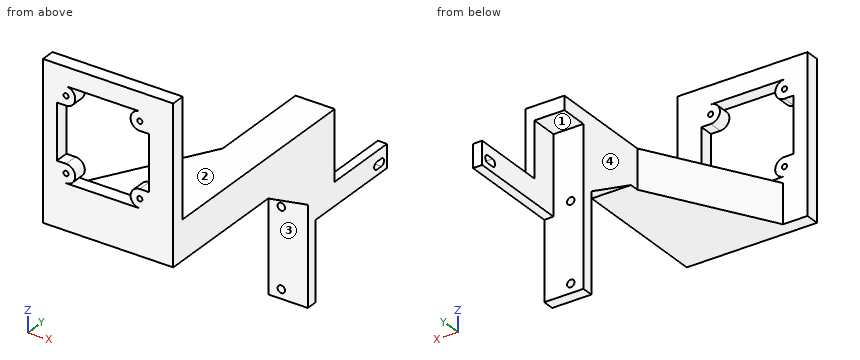
Autodesk Inventor part; units mm, degrees
ref_plane "YZ Plane" through (0, 0, 0) normal (1, 0, 0) x (0, 1, 0)
ref_plane "XZ Plane" through (0, 0, 0) normal (0, 1, 0) x (-1, 0, 0)
ref_plane "XY Plane" through (0, 0, 0) normal (0, 0, 1) x (1, 0, 0)
sketch "Sketch1" plane through (0, 0, 0) normal (0, 1, 0) x (-1, 0, 0)
  line L0 (0, 0) -> (13, 0)
  line L1 (13, 0) -> (13, -44)
  line L2 (13, -44) -> (0, -44)
  line L3 (0, -44) -> (0, 0)
  line L4 (13, 0) -> (13, -6)
  line L5 (13, -6) -> (7.5, -6)
  line L6 (7.5, -6) -> (7.5, -40)
  circle A0 centre (7.5, -6) radius 1.6
  circle A1 centre (7.5, -40) radius 1.6
  dimension "d0" = 13
  dimension "d1" = 44
  dimension "d2" = 6
  dimension "d3" = 5.5
  dimension "d4" = 34
  dimension "d5" = 3.2
  dimension "d6" = 3.2
extrude "Extrusion1" add sketch "Sketch1" along normal blind 5
sketch "Sketch2" plane through (0, 0, 0) normal (1, 0, 0) x (0, 0, -1)
  line L0 (0, 5) -> (44, 5)
  line L1 (0, 5) -> (44, 5)
  line L2 (44, 5) -> (44, 50)
  line L3 (44, 50) -> (0, 50)
  line L4 (0, 50) -> (0, 5)
  line L5 (0, 0) -> (44, 0)
  line L6 (44, 0) -> (44, 5)
  line L7 (44, 5) -> (0, 5)
  line L8 (0, 5) -> (0, 0)
  line L9 (0, 50) -> (10, 50)
  line L10 (10, 50) -> (10, 5)
  line L11 (10, 5) -> (0, 5)
  line L12 (0, 5) -> (0, 50)
  dimension "d9" = 44
  dimension "d10" = 45
  dimension "d11" = 10
extrude "Extrusion2" add sketch "Sketch2" along normal blind 4 contours L4 L3 L10 L0 | L0 L6 L5 L8
sketch "Sketch3" plane through (4, 0, 0) normal (1, 0, 0) x (0, 0, -1)
  line L0 (44, 5) -> (10, 5)
  line L1 (10, 5) -> (10, 45)
  line L2 (10, 5) -> (10, 50)
  line L3 (0, 50) -> (0, 5)
  line L4 (0, 45) -> (4.4, 45)
  line L5 (6, 45) -> (6, 46.5)
  line L6 (6, 45) -> (6, 43.5)
  line L7 (4.4, 46.5) -> (4.4, 43.5)
  line L8 (7.6, 46.5) -> (7.6, 43.5)
  arc A0 (5.4432, 45) -> (6, 44.9) centre (6, 46.5) ccw
  arc A1 (6.5568, 45) -> (4.4, 46.5) centre (6, 46.5) ccw
  line L9 (10, 45) -> (6.5568, 45)
  line L10 (5.4432, 45) -> (0, 45)
  arc A2 (6, 45.1) -> (5.4432, 45) centre (6, 43.5) ccw
  arc A3 (4.4, 43.5) -> (7.6, 43.5) centre (6, 43.5) ccw
  point P0 (0, 0)
  dimension "d14" = 40
  dimension "d15" = 6
  dimension "d16" = 1.5
  dimension "d17" = 1.5
extrude "Extrusion3" cut sketch "Sketch3" against normal blind 4 contours L6 A0 A2 L5 | A1 L9 L8 A3 L7 | L8 L9 A1
sketch "Sketch4" plane through (-13, 0, 0) normal (0, 0, 1) x (1, 0, 0)
  line L0 (0, 0) -> (17, 0)
  line L1 (17, 0) -> (17, 5)
  line L2 (0, 0) -> (17, 0)
  line L3 (17, 0) -> (17, 5)
  line L4 (17, 5) -> (0, 5)
  line L5 (0, 5) -> (0, 0)
  line L6 (13, 50) -> (13, 5)
  line L7 (17, 0) -> (13, 0)
  line L8 (13, 0) -> (13, 17)
  line L9 (13, 17) -> (17, 17)
  line L10 (17, 17) -> (17, 0)
  dimension "d22" = 17
extrude "Extrusion4" add sketch "Sketch4" along normal blind 30
sketch "Sketch5" plane through (0, 0, 0) normal (0, -1, 0) x (1, 0, 0)
  line L0 (-13, -44) -> (-13, 30)
  line L1 (-13, 30) -> (4, 30)
  line L2 (4, 30) -> (4, 13)
  line L3 (4, 13) -> (-13, 13)
  line L4 (-13, 13) -> (-13, 30)
  point P0 (0, 0)
  dimension "d25" = 17
  dimension "d26" = 17
extrude "Extrusion5" add sketch "Sketch5" along normal blind 85
sketch "Sketch7" plane through (0, -85, 0) normal (0, -1, 0) x (1, 0, 0)
  line L0 (4, 13) -> (-13, 13)
  line L1 (0, 30) -> (0, -10)
  line L2 (0, 13) -> (0, 30)
  line L3 (0, 30) -> (0, 52.6)
  circle A0 centre (-36, 52.6) radius 9
  line L4 (-36, 52.6) -> (-36, 36.6)
  line L5 (-36, 36.6) -> (-20, 36.6)
  line L6 (-36, 52.6) -> (-36, 68.6)
  line L7 (-36, 68.6) -> (-52, 68.6)
  line L8 (-52, 68.6) -> (-20, 68.6)
  line L9 (-20, 68.6) -> (-20, 36.6)
  line L10 (-20, 36.6) -> (-52, 36.6)
  line L11 (-52, 36.6) -> (-52, 68.6)
  circle A1 centre (-20, 68.6) radius 1.1
  circle A2 centre (-20, 36.6) radius 1.1
  circle A3 centre (-52, 36.6) radius 1.1
  circle A4 centre (-52, 68.6) radius 1.1
  circle A5 centre (-20, 68.6) radius 4
  circle A6 centre (-20, 36.6) radius 4
  line L12 (-52, 65.6) -> (-52, 70.6)
  line L13 (-52, 36.6) -> (-52, 42.6)
  circle A7 centre (-52, 68.6) radius 4
  circle A8 centre (-52, 36.6) radius 4
  point P0 (0, 0)
  point P1 (-20, 64.6)
  point P2 (-20, 40.6)
  dimension "d29" = 22.6
  dimension "d31" = 18
  dimension "d32" = 16
  dimension "d33" = 16
  dimension "d34" = 16
  dimension "d35" = 16
  dimension "d36" = 2.2
  dimension "d37" = 2.2
  dimension "d39" = 2.2
  dimension "d40" = 8
  dimension "d43" = 8
  dimension "d49" = 8
  dimension "d50" = 8
sketch "Sketch14" plane through (0, -85, 0) normal (0, -1, 0) x (1, 0, 0)
  line L0 (4, 13) -> (4, 30)
  line L1 (4, 13) -> (4, 52.6)
  line L2 (4, 52.6) -> (-26.5, 52.6)
  line L3 (-26.5, 52.6) -> (-26.5, 36.6)
  line L4 (-26.5, 36.6) -> (-10.5, 36.6)
  line L5 (-26.5, 52.6) -> (-42.5, 52.6)
  line L6 (-42.5, 52.6) -> (-42.5, 68.6)
  line L7 (-42.5, 68.6) -> (-10.5, 68.6)
  line L8 (-10.5, 68.6) -> (-10.5, 36.6)
  line L9 (-10.5, 36.6) -> (-42.5, 36.6)
  line L10 (-42.5, 36.6) -> (-42.5, 68.6)
  circle A0 centre (-42.5, 68.6) radius 1.1
  circle A1 centre (-10.5, 68.6) radius 1.1
  circle A2 centre (-10.5, 36.6) radius 1.1
  circle A3 centre (-42.5, 36.6) radius 1.1
  circle A4 centre (-42.5, 68.6) radius 4
  circle A5 centre (-10.5, 68.6) radius 4
  circle A6 centre (-10.5, 36.6) radius 4
  circle A7 centre (-42.5, 36.6) radius 4
  point P0 (0, 0)
  dimension "d91" = 39.6
  dimension "d92" = 30.5
  dimension "d93" = 16
  dimension "d94" = 16
  dimension "d95" = 16
  dimension "d96" = 16
  dimension "d97" = 2.2
  dimension "d98" = 2.2
  dimension "d99" = 2.2
  dimension "d100" = 2.2
  dimension "d101" = 8
  dimension "d102" = 8
  dimension "d103" = 8
  dimension "d104" = 8
extrude "Extrusion14" add sketch "Sketch14" against normal blind 6 contours A5 L7 A1 L8 | L8 A1 L7 A5 | A6 L4 A2 L8 | L8 A2 L4 A6 | A7 L10 A3 L9 | L9 A3 L10 A7 | A4 L7 A0 L6 | L6 A0 L7 A4
sketch "Sketch15" plane through (-10.5, -85, 68.6) normal (0, -1, 0) x (1, 0, 0)
  circle A0 centre (0, 0) radius 4
  line L0 (0, 4) -> (10, 4)
  line L1 (10, 4) -> (10, -4)
  line L2 (10, -4) -> (0, -4)
  line L3 (0, -4) -> (0, 4)
  circle A1 centre (0, -32) radius 4
  line L4 (0, -28) -> (10, -28)
  line L5 (10, -28) -> (10, -36)
  line L6 (10, -36) -> (0, -36)
  line L7 (0, -36) -> (0, -28)
  circle A2 centre (-32, -32) radius 4
  line L8 (-32, -36) -> (-42, -36)
  line L9 (-42, -36) -> (-42, -28)
  line L10 (-42, -28) -> (-32, -28)
  line L11 (-32, -28) -> (-32, -36)
  circle A3 centre (-32, 0) radius 4
  line L12 (-32, -4) -> (-42, -4)
  line L13 (-42, -4) -> (-42, 4)
  line L14 (-42, 4) -> (-32, 4)
  line L15 (-32, 4) -> (-32, -4)
  line L16 (-42, 4) -> (-36, 4)
  line L17 (-36, 4) -> (-36, -36)
  line L18 (-36, -36) -> (-42, -36)
  line L19 (-42, -36) -> (-42, 4)
  line L20 (10, 4) -> (4, 4)
  line L21 (4, 4) -> (4, -36)
  line L22 (4, -36) -> (10, -36)
  line L23 (10, -36) -> (10, 4)
  point P0 (10.5, -68.6)
  point P1 (-36, -4)
  point P2 (-32, 4)
  point P3 (-42, -4)
  point P4 (-36, -28)
  point P5 (0, -4)
  point P6 (4, -4)
  point P7 (4, -28)
  point P8 (10, -4)
  dimension "d107" = 10
  dimension "d108" = 8
  dimension "d109" = 10
  dimension "d110" = 8
  dimension "d111" = 10
  dimension "d112" = 8
  dimension "d113" = 10
  dimension "d114" = 8
  dimension "d115" = 6
  dimension "d116" = 6
extrude "Extrusion15" add sketch "Sketch15" against normal blind 6 contours L21 L2 A0 | A0 L0 L21 | L21 L0 L1 L2 | L2 L23 L4 L21 | L21 A1 L4 | L4 L5 L6 L21 | L21 L6 A1 | A2 L17 L10 | L8 L17 A2 | L17 L8 L9 L10 | L10 L19 L12 L17 | L17 A3 L12 | L12 L13 L14 L17 | L17 L14 A3
sketch "Sketch16" plane through (0, -85, 0) normal (0, -1, 0) x (1, 0, 0)
  line L0 (-0.5, 72.6) -> (-0.5, 32.6)
  line L1 (-0.5, 72.6) -> (-52.5, 72.6)
  line L2 (-52.5, 72.6) -> (-52.5, 80.6)
  line L3 (-52.5, 80.6) -> (-0.5, 80.6)
  line L4 (-0.5, 80.6) -> (-0.5, 72.6)
  line L5 (-0.5, 32.6) -> (-10.5, 32.6)
  line L6 (-0.5, 32.6) -> (-52.5, 32.6)
  line L7 (-52.5, 32.6) -> (-52.5, 24.6)
  line L8 (-52.5, 24.6) -> (-0.5, 24.6)
  line L9 (-0.5, 24.6) -> (-0.5, 32.6)
  point P0 (0, 0)
  dimension "d119" = 8
  dimension "d120" = 8
extrude "Extrusion16" add sketch "Sketch16" against normal blind 6
sketch "Sketch17" plane through (0, -79, 0) normal (0, 1, 0) x (1, 0, 0)
  line L0 (-0.5, -80.6) -> (-0.5, -30)
  line L1 (4, -30) -> (0, -30)
  line L2 (-0.5, -80.6) -> (4, -80.6)
  line L3 (4, -80.6) -> (4, -30)
  line L4 (4, -30) -> (-0.5, -30)
  line L5 (-0.5, -30) -> (-0.5, -80.6)
  line L6 (-52.5, -24.6) -> (-52.5, -80.6)
  line L7 (-52.5, -24.6) -> (-13, -24.6)
  line L8 (-13, -24.6) -> (-13, -13)
  line L9 (-13, -13) -> (-52.5, -13)
  line L10 (-52.5, -13) -> (-52.5, -24.6)
  point P0 (0, 0)
extrude "Extrusion17" add sketch "Sketch17" against normal blind 6
chamfer "Chamfer4" distance 50 angle 30 1 edges at (-13, -79, 21.5) measured on face at (-13, -24.6667, 24.3333)
chamfer "Chamfer5" distance 25 angle 30 1 edges at (-4.5, 0, 13) measured on face at (-16.9558, -64.3333, 13)
sketch "Sketch19" plane through (-13, 0, 30) normal (0, 0, 1) x (1, 0, 0)
  line L0 (13, 17) -> (13, 5)
  line L1 (0, 0) -> (0, 5)
  line L2 (13, 17) -> (0, 17)
  line L3 (0, 17) -> (0, 5)
  line L4 (0, 5) -> (13, 5)
  line L5 (13, 5) -> (13, 17)
  point P0 (13, 0)
extrude "Extrusion18" add sketch "Sketch19" against normal blind 6
properties part number "camera_mount_v1"
Here's how the part is built. I have some questions about the finished solid (model axes, mm). Face numbers are marked on the shaded views. A direction names the side the tool comes from. Coordinates: 2 decimals unless noted, no trailing zeros. Loops run counter-clockwise (first coordinate to the right, second up) from the corner with the lowest first, then second, coordinate; pieces in that order, holes last. Notation, with made-up numbers: (1.25, 50.25) - (6.25, 50.25) arc R17 ccw to (6.25, 59.25) - close; hole circle Ø2 at (14, -20.75). An arc over 180 degrees is marked (long way). Return JSON: item names as keys, results as strings. Group by question number.
Item 1: If we section it at A-A on z = -6: Write out the boundary of the cut face in (x, y), and give its area (3 significant figures).
Item 2: On a 3-axis mill with a long thin cutter (end or side, diameter ignored), from which of +Z, -Z, +X, -X, +Y, -Y can I reach the whole of each face in a straight line? I mean the marked faces 1, 2, 3 and 4. Say none if no direction works.
Item 3: Will these pins go through, and if not, where does the flat tip stop? P1, Ø12, axis at x = -11.5, y = -70.5, coming from the -Z side; P2, Ø5, axis at x = -5, z = 13.5, coming from the +Y side; P3, Ø3.5, axis at x = -6.5, y = 10.5, coming from the -Z side.
Item 4: If we section it at C-C on x = -3: Write out the boundary of the cut face in (y, z), and give its area (3 significant figures).
Item 5: If we section it at B-B on z = -40: Write out the boundary of the cut face in (x, y), and give its area (3 significant figures).
Item 6: If we section it at D-D on x = -16.5: Write out the boundary of the cut face in (y, z), and give its area (3 significant figures).
Item 7: I need wall thicknesses on line 1 (Z direction, x = -7.5, y = 2.5); line 2 (X direction, y = -82.8, z = 36.6); line 3 (X direction, y = -81, z = 36). Which ranges of each line are inside material? Lowest first, please. Write a range as from..to.
Calculated:
{
 "1": {"outline": "(-13, 0) - (-9.1, 0) - (-9.1, 5) - (-13, 5) - close; (-5.9, 0) - (4, 0) - (4, 41.9) - (0, 41.9) - (0, 5) - (-5.9, 5) - close; (0, 48.1) - (4, 48.1) - (4, 50) - (0, 50) - close", "area": "224 mm^2"},
 "2": {"face 1": "-Z, -X, +Y", "face 2": "+Z, +X, -X, +Y", "face 3": "-Z, +X, -X, -Y", "face 4": "+Z, -Z, -X, +Y"},
 "3": {"P1": "stops at z = 13", "P2": "stops at y = 5", "P3": "stops at z = 24"},
 "4": {"outline": "(-85, 13) - (-25, 13) - (0, -1.43) - (0, -44) - (5, -44) - (5, 24) - (17, 24) - (17, 30) - (-79, 30) - (-79, 80.6) - (-85, 80.6) - close", "area": "2,370 mm^2"},
 "5": {"outline": "(-13, 0) - (-9.1, 0) - (-9.1, 5) - (-13, 5) - close; (-5.9, 0) - (4, 0) - (4, 5) - (-5.9, 5) - close", "area": "69.0 mm^2"},
 "6": {"outline": "(-85, 13) - (-35.06, 13) - (-35.06, 30) - (-79, 30) - (-79, 32.6) - (-85, 32.6) - close; (-85, 72.6) - (-79, 72.6) - (-79, 80.6) - (-85, 80.6) - close", "area": "913 mm^2"},
 "7": {"line 1": "z = -44..-41.6, -38.4..-7.6, -4.4..30", "line 2": "x = -52.5..-43.6, -41.4..-38.5, -14.5..-11.6, -9.4..4", "line 3": "x = -52.5..-43.42, -41.58..-38.55, -14.45..-11.42, -9.58..4"}
}
